Part model, mm, in its own coordinate system. Face numbers are marked on the shaded views. A direction names the side the tool comes from. Round coordinates to 2 decimals unless told otherwise and drop trailing zeros. Order: outer loops, then holes, each group sorted by start corner. A loop starts at its lowest first (then second) coordinate and runs counter-clockwise, first axis right, second up. Notation, with made-up numbers: M 80.5,38 L 93.5,38 A18 cw 93.5,65 Z; hole C 9,13 d4. An arc over 180 degrees is marked long. Write each question's results on one line, items separated by ' | '. Start each with the question number.
1. Band-saw the part on C-C, the plane y = -27.94. List the corners of the cut face in (x, z), then the cut area to 3 significant figures.
2. Two-plate mould, pull along X, no slides. Class the marked faces 1, 2 and 3: +X half, -X half, draft (parallel to the pull), parting line (faces both ways), or undercut.
3. Which spindle directions (+Z, -Z, +X, -X, +Y, -Y) get a long thin tool onto all of the face, cutting with end or side? Do the marked faces 4, 5 and 6. Say none if no direction does.
4. Band-saw the part on B-B, the plane x = 101.6. List the corners of the cut face in (y, z) (3 decimals).
5. Band-saw the part on A-A, the plane z = 38.1. Give the number of separate pieces and of enclosed holes in the cut face, then the cut area to 3 significant figures.
6. Band-saw the part on D-D, the plane z = 31.5. List the corners of the cut face in (x, y) (3 decimals).
7. Probe L1, parallel to X at y = -27.5, z = 23.5; L2, parallel to X at y = -35.5, z = 20.5; L3, parallel to Y at x = 98, z = 6 (3 decimals). List the from-to ranges inside material, lowest first. Write a range as [from, to].
8. Drop flat-ended pins along their axis: pin 1 Ø6.5 at (x, z) = (9.652, 38.1) entering from +Y; pin 2 Ø15.5 at (x, z) = (146.5, 19) entering from -Y; pin 3 Ø12 at (x, z) = (135, 14.5) entering from -Y. Give the stop position or say it passes through.
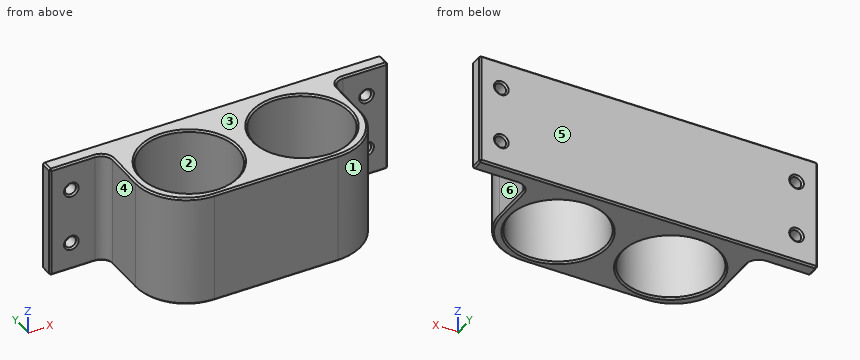
```python
from build123d import *

# Parameters (mm, degrees)
F0_W     = 25.4
F0_H     = 50.8
F0_R     = 2.54
F0_W_2   = 50.8
F1_DEPTH = 6.35
F2_DEPTH = 52.705
F3_R     = 5.08
F4_R     = 21.59
F5_DEPTH = 50.801
F6_R     = 22.86
F7_SIZE  = 0.762


with BuildPart() as f1:
    # F0 (on Front) → F1 (new body)
    with BuildSketch(Plane.XZ):
        with Locations((12.7, 25.4)):
            Rectangle(F0_W, F0_H)
        with Locations((9.652, 12.7)):
            Circle(F0_R, mode=Mode.SUBTRACT)
        with Locations((9.652, 38.1)):
            Circle(F0_R, mode=Mode.SUBTRACT)
        with Locations((139.7, 25.4)):
            Rectangle(F0_W, F0_H)
        with Locations((142.748, 12.7)):
            Circle(F0_R, mode=Mode.SUBTRACT)
        with Locations((142.748, 38.1)):
            Circle(F0_R, mode=Mode.SUBTRACT)
        with Locations((50.8, 25.4)):
            Rectangle(F0_W_2, F0_H)
        with Locations((101.6, 25.4)):
            Rectangle(F0_W_2, F0_H)
    extrude(amount=F1_DEPTH)

    # F0 (on Front) → F2 (join)
    with BuildSketch(Plane.XZ):
        with Locations((50.8, 25.4)):
            Rectangle(F0_W_2, F0_H)
        with Locations((101.6, 25.4)):
            Rectangle(F0_W_2, F0_H)
    extrude(amount=F2_DEPTH)

    # F3
    f3_edges = [f1.edges().sort_by_distance(p)[0] for p in [
        (127, -6.35, 25.4),
        (25.4, -6.35, 25.4),
    ]]
    fillet(f3_edges, radius=F3_R)

    # F4 (on face) → F5 (cut, through all)
    with BuildSketch(Plane.XY.offset(50.8)):
        with Locations((50.8, -27.94)):
            Circle(F4_R)
        with Locations((101.6, -27.94)):
            Circle(F4_R)
    extrude(amount=-F5_DEPTH, mode=Mode.SUBTRACT)

    # F6
    f6_edges = [f1.edges().sort_by_distance(p)[0] for p in [
        (127, -52.705, 25.4),
        (25.4, -52.705, 25.4),
    ]]
    fillet(f6_edges, radius=F6_R)

    # F7
    f7_edges = [f1.edges().sort_by_distance(p)[0] for p in [
        (127, -20.6375, 50.8),
        (120.304461, -46.009461, 50.8),
        (128.487898, -7.837898, 50.8),
        (76.2, -52.705, 50.8),
        (142.24, -6.35, 50.8),
        (32.095539, -46.009461, 50.8),
        (152.4, -3.175, 50.8),
        (25.4, -20.6375, 50.8),
        (76.2, 0, 50.8),
        (23.912102, -7.837898, 50.8),
        (0, -3.175, 50.8),
        (10.16, -6.35, 50.8),
        (80.01, -27.94, 50.8),
        (29.21, -27.94, 50.8),
        (20.32, -6.35, 25.4),
        (0, -6.35, 25.4),
        (10.16, -6.35, 0),
        (7.112, -6.35, 12.7),
        (7.112, -6.35, 38.1),
        (132.08, -6.35, 25.4),
        (152.4, -6.35, 25.4),
        (142.24, -6.35, 0),
        (140.208, -6.35, 12.7),
        (140.208, -6.35, 38.1),
        (25.4, -20.6375, 0),
        (32.095539, -46.009461, 0),
        (23.912102, -7.837898, 0),
        (76.2, -52.705, 0),
        (120.304461, -46.009461, 0),
        (0, -3.175, 0),
        (127, -20.6375, 0),
        (76.2, 0, 0),
        (128.487898, -7.837898, 0),
        (152.4, -3.175, 0),
        (29.21, -27.94, 0),
        (80.01, -27.94, 0),
        (0, 0, 25.4),
        (152.4, 0, 25.4),
        (7.112, 0, 12.7),
        (7.112, 0, 38.1),
        (140.208, 0, 38.1),
        (140.208, 0, 12.7),
    ]]
    chamfer(f7_edges, length=F7_SIZE)


solid = f1.part
```
Solution:
1) outline: M 25.4,0.76 L 26.16,0 L 28.45,0 L 29.21,0.76 L 29.21,50.04 L 28.45,50.8 L 26.16,50.8 L 25.4,50.04 Z; M 72.39,0.76 L 73.15,0 L 79.25,0 L 80.01,0.76 L 80.01,50.04 L 79.25,50.8 L 73.15,50.8 L 72.39,50.04 Z; M 123.19,0.76 L 123.95,0 L 126.24,0 L 127,0.76 L 127,50.04 L 126.24,50.8 L 123.95,50.8 L 123.19,50.04 Z | area: 771 mm^2
2) face 1: +X half | face 2: undercut | face 3: draft
3) face 4: +Z, -Z, -X, -Y | face 5: +Z, -Z, +X, -X, +Y | face 6: +Z, -Z, +X, -Y
4) outline: M -52.705,0.762 L -51.943,0 L -50.292,0 L -49.53,0.762 L -49.53,50.038 L -50.292,50.8 L -51.943,50.8 L -52.705,50.038 Z; M -6.35,0.762 L -5.588,0 L -0.762,0 L 0,0.762 L 0,50.038 L -0.762,50.8 L -5.588,50.8 L -6.35,50.038 Z
5) separate pieces: 3 | enclosed holes: 2 | area: 2,470 mm^2
6) outline: M 0,-5.588 L 0.762,-6.35 L 20.32,-6.35 A5.08 cw 25.4,-11.43 L 25.4,-29.845 A22.86 ccw 48.26,-52.705 L 104.14,-52.705 A22.86 ccw 127,-29.845 L 127,-11.43 A5.08 cw 132.08,-6.35 L 151.638,-6.35 L 152.4,-5.588 L 152.4,-0.762 L 151.638,0 L 0.762,0 L 0,-0.762 Z; hole C 50.8,-27.94 d43.18; hole C 101.6,-27.94 d43.18
7) L1: [25.4, 29.21], [72.39, 80.01], [123.19, 127] | L2: [26.11, 30.58], [71.02, 81.38], [121.82, 126.29] | L3: [-52.705, -49.228], [-6.652, 0]
8) pin 1: y = -0.05 | pin 2: y = -6.35 | pin 3: y = -7.39
